Geometry check sheet. Reference: the model listing, model coordinates, mm. A direction names the side the tool comes from. Coordinates: 2 decimals unless noted, no trailing zeros. Loops run counter-clockwise (first coordinate to the right, second up) from the corner with the lowest first, then second, coordinate; pieces in that order, holes last.
from build123d import *

# Parameters (mm, degrees)
SKETCH2_W           = 70
SKETCH2_H           = 140
BOSS_EXTRUDE1_DEPTH = 15
SKETCH7_W           = 70
SKETCH7_H           = 125
CUT_EXTRUDE4_DEPTH  = 12.5
SKETCH8_W           = 5
SKETCH8_H           = 5
CUT_EXTRUDE5_DEPTH  = 7
SKETCH6_R           = 8.4
CUT_EXTRUDE2_DEPTH  = 16
SKETCH9_OUTSIDE_W   = 103.448
SKETCH9_OUTSIDE_H   = 173.448
SKETCH9_OUTSIDE_W_2 = 60
SKETCH9_OUTSIDE_H_2 = 140
CUT_EXTRUDE6_DEPTH  = 15
SKETCH10_W          = 60
SKETCH10_H          = 2
CUT_EXTRUDE7_DEPTH  = 140
SKETCH11_W          = 5
SKETCH11_H          = 5
BOSS_EXTRUDE2_DEPTH = 30
SKETCH12_W          = 5
SKETCH12_H          = 5
BOSS_EXTRUDE3_DEPTH = 20
SKETCH13_W          = 5
SKETCH13_H          = 5
BOSS_EXTRUDE4_DEPTH = 10
SKETCH15_W          = 5
SKETCH15_H          = 5
BOSS_EXTRUDE5_DEPTH = 20
SKETCH16_W          = 5
SKETCH16_H          = 5
BOSS_EXTRUDE6_DEPTH = 10


with BuildPart() as part:
    # Sketch2 → Boss-Extrude1 (new body)
    with BuildSketch(Plane.XY):
        with Locations((35, 70)):
            Rectangle(SKETCH2_W, SKETCH2_H)
    extrude(amount=BOSS_EXTRUDE1_DEPTH)

    # Sketch7 → Cut-Extrude4 (cut)
    with BuildSketch(Plane.XY.offset(15)):
        with Locations((35, 70)):
            Rectangle(SKETCH7_W, SKETCH7_H)
    extrude(amount=-CUT_EXTRUDE4_DEPTH, mode=Mode.SUBTRACT)

    # Sketch8 → Cut-Extrude5 (cut)
    with BuildSketch(Plane.XY.offset(15)):
        with Locations((12.5, 136)):
            Rectangle(SKETCH8_W, SKETCH8_H)
        with Locations((57.5, 136)):
            Rectangle(SKETCH8_W, SKETCH8_H)
        with Locations((12.5, 4)):
            Rectangle(SKETCH8_W, SKETCH8_H)
        with Locations((57.5, 4)):
            Rectangle(SKETCH8_W, SKETCH8_H)
    extrude(amount=-CUT_EXTRUDE5_DEPTH, mode=Mode.SUBTRACT)

    # Sketch6 → Cut-Extrude2 (cut, through all)
    with BuildSketch(Plane(origin=(0, 0, 0), x_dir=(-1, 0, 0), z_dir=(0, 0, -1))):
        with Locations((-35, 70)):
            Circle(SKETCH6_R)
    extrude(amount=-CUT_EXTRUDE2_DEPTH, mode=Mode.SUBTRACT)

    # Sketch9 outside → Cut-Extrude6 (cut)
    with BuildSketch(Plane(origin=(0, 0, 0), x_dir=(-1, 0, 0), z_dir=(0, 0, -1))):
        with Locations((-35, 70)):
            Rectangle(SKETCH9_OUTSIDE_W, SKETCH9_OUTSIDE_H)
        with Locations((-35, 70)):
            Rectangle(SKETCH9_OUTSIDE_W_2, SKETCH9_OUTSIDE_H_2, mode=Mode.SUBTRACT)
    extrude(amount=-CUT_EXTRUDE6_DEPTH, mode=Mode.SUBTRACT)

    # Sketch10 → Cut-Extrude7 (cut)
    with BuildSketch(Plane(origin=(0, 140, 0), x_dir=(1, 0, 0), z_dir=(0, 1, 0))):
        with Locations((35, -14)):
            Rectangle(SKETCH10_W, SKETCH10_H)
    extrude(amount=-CUT_EXTRUDE7_DEPTH, mode=Mode.SUBTRACT)

    # Sketch11 → Boss-Extrude2 (add)
    with BuildSketch(Plane.XZ):
        with Locations((47.5, 8.5)):
            Rectangle(SKETCH11_W, SKETCH11_H)
        with Locations((22.5, 8.5)):
            Rectangle(SKETCH11_W, SKETCH11_H)
    extrude(amount=BOSS_EXTRUDE2_DEPTH)

    # Sketch12 → Boss-Extrude3 (add)
    with BuildSketch(Plane.XY.offset(11)):
        with Locations((22.5, -27.5)):
            Rectangle(SKETCH12_W, SKETCH12_H)
    extrude(amount=BOSS_EXTRUDE3_DEPTH)

    # Sketch13 → Boss-Extrude4 (add)
    with BuildSketch(Plane(origin=(0, -25, 0), x_dir=(1, 0, 0), z_dir=(0, 1, 0))):
        with Locations((22.5, -28.5)):
            Rectangle(SKETCH13_W, SKETCH13_H)
    extrude(amount=BOSS_EXTRUDE4_DEPTH)

    # Sketch15 → Boss-Extrude5 (add)
    with BuildSketch(Plane.XY.offset(11)):
        with Locations((47.5, -27.5)):
            Rectangle(SKETCH15_W, SKETCH15_H)
    extrude(amount=BOSS_EXTRUDE5_DEPTH)

    # Sketch16 → Boss-Extrude6 (add)
    with BuildSketch(Plane(origin=(0, -25, 0), x_dir=(1, 0, 0), z_dir=(0, 1, 0))):
        with Locations((47.5, -28.5)):
            Rectangle(SKETCH16_W, SKETCH16_H)
    extrude(amount=BOSS_EXTRUDE6_DEPTH)


solid = part.part
1) Mould release check, pull along X, two halves, no side actions. Record for faces 6 (the flat face through (45, -25.2, 15.9)), 7 (the flat face through (5, 64, 2)), 8 (the flat face through (22, -25, 18)), 9 (the flat face through (12, 133.5, 11)): +X half, -X half, draft (parallel to the pull), parting line (faces both ways), or undercut.
Data:
face 6: undercut
face 7: -X half
face 8: draft
face 9: undercut
2) Section check C-C on z = 20. Record the cut outline in (x, y), and give its area (3 significant figures).
Data:
outline: (20, -30) - (25, -30) - (25, -25) - (20, -25) - close; (45, -30) - (50, -30) - (50, -25) - (45, -25) - close
area: 50.0 mm2
3) Depth check by flat-ended pin: pin 1 (2.5 mm diameter, centred on x = 23.5, y = -12.5, fed in from +Z); pin 2 (8 mm diameter, centred on x = 15.5, y = 96.5, fed in from -Z); pin 3 (5.5 mm diameter, centred on x = 23.5, y = -21.5, fed in from -Z); pin 4 (5.5 mm diameter, centred on x = 58.5, z = 10, fed in from -Y). Enter the tip coordinate at first touch or a pass-through.
Data:
pin 1: stops at z = 11
pin 2: stops at z = 0
pin 3: stops at z = 6
pin 4: stops at y = 0
4) Access from +Z, -Z, +X, -X, +Y, -Y to the whole of each face (thin tool, end or side, straight path). Record for faces 1 (the flat face through (35, 4, 13)), 2 (the flat face through (57, 133.5, 11)), 3 (the flat face through (22, -20, 26)), 4 (the flat face through (22, -12, 11)), 5 (the flat face through (35, 132.5, 8)).
Data:
face 1: +Z, +X, -X, +Y
face 2: +Z
face 3: +X, -X, +Y
face 4: +X, -X
face 5: +Z, +X, -X
5) Section check A-A on y = 70. Record the cut outline in (x, z), and give its area (3 significant figures).
Data:
outline: (5, 0) - (26.6, 0) - (26.6, 2.5) - (5, 2.5) - close; (43.4, 0) - (65, 0) - (65, 2.5) - (43.4, 2.5) - close
area: 108 mm2
6) Material ranges on probe 1 along Y at (x, z) = (35, 1.65); probe 2 along Z at (x, y) = (53.5, 78); probe 3 along Y at (x, z) = (9.5, 9.5), recorded low to high.
Data:
probe 1: y = 0 to 61.6, 78.4 to 140
probe 2: z = 0 to 2.5
probe 3: y = 0 to 7.5, 132.5 to 140
7) Section check B-B on x = 35. Record the cut outline in (y, z), and give its area (4 significant figures).
Data:
outline: (0, 0) - (61.6, 0) - (61.6, 2.5) - (7.5, 2.5) - (7.5, 13) - (0, 13) - close; (78.4, 0) - (140, 0) - (140, 13) - (132.5, 13) - (132.5, 2.5) - (78.4, 2.5) - close
area: 465.5 mm2
8) Section check D-D on x = 13. Record the cut outline in (y, z).
Data:
outline: (0, 0) - (140, 0) - (140, 13) - (138.5, 13) - (138.5, 8) - (133.5, 8) - (133.5, 13) - (132.5, 13) - (132.5, 2.5) - (7.5, 2.5) - (7.5, 13) - (6.5, 13) - (6.5, 8) - (1.5, 8) - (1.5, 13) - (0, 13) - close
